Here's how the part is built. I have some questions about the finished solid (model axes, mm). Give positions to 0.01 mm unless a question says otherwise; leave off trailing zeros. Order: outer loops, then holes, each group sorted by start corner. A loop starts at its lowest first (then second) coordinate and runs counter-clockwise, first axis right, second up. Notation, with made-up numbers: M 72.25,66.5 L 107.25,66.5 A38 cw 107.25,105.5 Z; hole C 32,-39 d2. An arc over 180 degrees is marked long. Use CSV: the item, a comma, the result in double quotes. Start each with the question number.
```python
from build123d import *

# Parameters (mm, degrees)
SKETCH1_R           = 2.5
EXTRUDE_1_DEPTH     = 210
CUT_EXTRUDE_1_DEPTH = 212.187120819


with BuildPart() as part:
    # Sketch1 → 凸台-拉伸1 (new body)
    with BuildSketch(Plane.XY):
        with BuildLine():
            Line((-3.6, 10), (-3.6, 9.5))
            Line((-3.6, 9.5), (-3.1, 9.5))
            Line((-3.1, 9.5), (-3.1, 8.5))
            Line((-3.1, 8.5), (-5.5, 8.5))
            Line((-5.5, 8.5), (-5.5, 6.65))
            Line((-5.5, 6.65), (-2.75, 3.9))
            Line((-2.75, 3.9), (2.75, 3.9))
            Line((2.75, 3.9), (5.5, 6.65))
            Line((5.5, 6.65), (5.5, 8.5))
            Line((5.5, 8.5), (3.1, 8.5))
            Line((3.1, 8.5), (3.1, 9.5))
            Line((3.1, 9.5), (3.6, 9.5))
            Line((3.6, 9.5), (3.6, 10))
            Line((3.6, 10), (8.5, 10))
            ThreePointArc((8.5, 10), (9.560660172, 9.560660172), (10, 8.5))
            Line((10, 8.5), (10, 3.6))
            Line((10, 3.6), (9.5, 3.6))
            Line((9.5, 3.6), (9.5, 3.1))
            Line((9.5, 3.1), (8.5, 3.1))
            Line((8.5, 3.1), (8.5, 5.5))
            Line((8.5, 5.5), (6.65, 5.5))
            Line((6.65, 5.5), (3.9, 2.75))
            Line((3.9, 2.75), (3.9, -2.75))
            Line((3.9, -2.75), (6.65, -5.5))
            Line((6.65, -5.5), (8.5, -5.5))
            Line((8.5, -5.5), (8.5, -3.1))
            Line((8.5, -3.1), (9.5, -3.1))
            Line((9.5, -3.1), (9.5, -3.6))
            Line((9.5, -3.6), (10, -3.6))
            Line((10, -3.6), (10, -8.5))
            ThreePointArc((10, -8.5), (9.560660172, -9.560660172), (8.5, -10))
            Line((8.5, -10), (3.6, -10))
            Line((3.6, -10), (3.6, -9.5))
            Line((3.6, -9.5), (3.1, -9.5))
            Line((3.1, -9.5), (3.1, -8.5))
            Line((3.1, -8.5), (5.5, -8.5))
            Line((5.5, -8.5), (5.5, -6.65))
            Line((5.5, -6.65), (2.75, -3.9))
            Line((2.75, -3.9), (-2.75, -3.9))
            Line((-2.75, -3.9), (-5.5, -6.65))
            Line((-5.5, -6.65), (-5.5, -8.5))
            Line((-5.5, -8.5), (-3.1, -8.5))
            Line((-3.1, -8.5), (-3.1, -9.5))
            Line((-3.1, -9.5), (-3.6, -9.5))
            Line((-3.6, -9.5), (-3.6, -10))
            Line((-3.6, -10), (-8.5, -10))
            ThreePointArc((-8.5, -10), (-9.560660172, -9.560660172), (-10, -8.5))
            Line((-10, -8.5), (-10, -3.6))
            Line((-10, -3.6), (-9.5, -3.6))
            Line((-9.5, -3.6), (-9.5, -3.1))
            Line((-9.5, -3.1), (-8.5, -3.1))
            Line((-8.5, -3.1), (-8.5, -5.5))
            Line((-8.5, -5.5), (-6.65, -5.5))
            Line((-6.65, -5.5), (-3.9, -2.75))
            Line((-3.9, -2.75), (-3.9, 2.75))
            Line((-3.9, 2.75), (-6.65, 5.5))
            Line((-6.65, 5.5), (-8.5, 5.5))
            Line((-8.5, 5.5), (-8.5, 3.1))
            Line((-8.5, 3.1), (-9.5, 3.1))
            Line((-9.5, 3.1), (-9.5, 3.6))
            Line((-9.5, 3.6), (-10, 3.6))
            Line((-10, 3.6), (-10, 8.5))
            ThreePointArc((-10, 8.5), (-9.560660172, 9.560660172), (-8.5, 10))
            Line((-8.5, 10), (-3.6, 10))
        make_face()
        Circle(SKETCH1_R, mode=Mode.SUBTRACT)
    extrude(amount=EXTRUDE_1_DEPTH)

    # 草图1 → 切除-拉伸1 (cut, through all)
    with BuildSketch(Plane(origin=(0, 10, 0), x_dir=(1, 0, 0), z_dir=(0, 1, 0))):
        Polygon((-9.86868981, -210), (10.13131019, -210), (10.13131019, -190), align=None)
        Polygon((-9.910928713, 0), (10.089071287, 0), (10.089071287, -20), align=None)
    extrude(amount=-CUT_EXTRUDE_1_DEPTH, mode=Mode.SUBTRACT)


solid = part.part
```
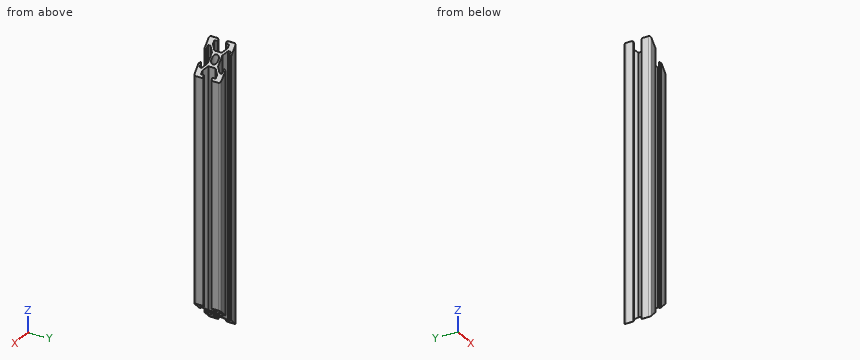
Q1. For P1, Ø2, axis at y = 2.5, z = 168.5, coming from the -X side; P2, Ø6, axis at x = -2, y = 4.5, coming from the +Z side; P3, Ø1.5, axis at x = 3, y = 8, coming from the -Z side; P4, Ø1.1, axis at y = 9, z = 118, coming from the +X side, each with a flat end and sliding along its axis, tell me the tip position at first contact or that it passes through.
Q2. Imagine slicing it at B-B, the plane x = 0. Please give me the cut outline in (y, z).
Q3. Imagine slicing it at A-A, the plane y = 0. Please give me the cut outline in (x, z).
Q4. I need wall thicknesses on line 1 (Y direction, x = 0, z = 137.5); line 2 (Y direction, x = -4.5, z = 174). Which ranges of each line are inside material? Lowest first, please. Write a range as [from, to].
Reply:
1,P1,"stops at x = -9.5"
1,P2,"stops at z = 205.13"
1,P3,"stops at z = 13.01"
1,P4,"stops at x = 10"
2,outline,"M -3.9,9.91 L -2.5,9.91 L -2.5,200.13 L -3.9,200.13 Z; M 2.5,9.91 L 3.9,9.91 L 3.9,200.13 L 2.5,200.13 Z"
3,outline,"M -3.9,6.01 L -2.5,7.41 L -2.5,202.63 L -3.9,204.03 Z; M 2.5,12.41 L 3.9,13.81 L 3.9,196.23 L 2.5,197.63 Z"
4,line 1,"y = [-3.9, -2.5], [2.5, 3.9]"
4,line 2,"y = [-10, -8.5], [-5.65, -3.35], [3.35, 5.65], [8.5, 10]"
